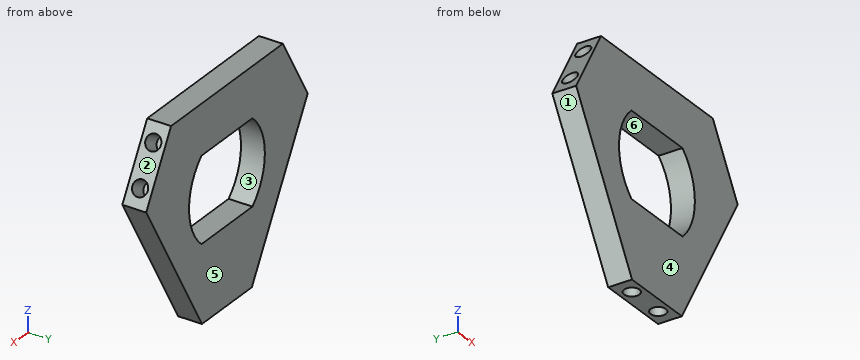
```python
from build123d import *

# Parameters (mm, degrees)
CROQUIS1_W              = 57.5
CROQUIS1_H              = 42.5
SALIENTE_EXTRUIR1_DEPTH = 12
CROQUIS7_R              = 46.25
CROQUIS7_R_2            = 28.75
SALIENTE_EXTRUIR2_DEPTH = 12
CROQUIS8_R              = 3.875
CORTAR_EXTRUIR1_DEPTH   = 10
MATRIZC1_COUNT          = 3


with BuildPart() as part:
    # Croquis1 → Saliente-Extruir1 (new body)
    with BuildSketch(Plane(origin=(0, 0, 0), x_dir=(1, 0, 0), z_dir=(0, 1, 0))):
        Polygon((-18.886751346, 59.787187079), (-61.220598504, -13.537187079), (-42.333847158, -46.25), (42.333847158, -46.25), (61.220598504, -13.537187079), (18.886751346, 59.787187079), align=None)
        Rectangle(CROQUIS1_W, CROQUIS1_H, mode=Mode.SUBTRACT)
    extrude(amount=SALIENTE_EXTRUIR1_DEPTH)

    # Croquis7 → Saliente-Extruir2 (add)
    with BuildSketch(Plane(origin=(0, 0, 0), x_dir=(1, 0, 0), z_dir=(0, 1, 0))):
        Circle(CROQUIS7_R)
        Circle(CROQUIS7_R_2, mode=Mode.SUBTRACT)
    extrude(amount=SALIENTE_EXTRUIR2_DEPTH)

    # Croquis8 → Cortar-Extruir1 (cut)
    with BuildSketch(Plane(origin=(51.777222831, 0, 29.893593539), x_dir=(0.5, 0, -0.866025404), z_dir=(0.866025404, 0, 0.5))):
        with Locations((-10, 6)):
            Circle(CROQUIS8_R)
        with Locations((10, 6)):
            Circle(CROQUIS8_R)
    cortar_extruir1 = extrude(amount=-CORTAR_EXTRUIR1_DEPTH, mode=Mode.SUBTRACT)

    # MatrizC1: Cortar-Extruir1 ×3 about axis
    matrizc1_axis = Axis((0, 0, 0), (0, 1, 0))
    for i in range(1, MATRIZC1_COUNT):
        add(cortar_extruir1.rotate(matrizc1_axis, i * 360 / MATRIZC1_COUNT), mode=Mode.SUBTRACT)


solid = part.part
```
Geometry check sheet. Reference: the model listing, model coordinates, mm. Face numbers are marked on the shaded views. A direction names the side the tool comes from. Coordinates: 2 decimals unless noted, no trailing zeros. Order: outer loops, then holes, each group sorted by start corner. A loop starts at its lowest first (then second) coordinate and runs counter-clockwise, first axis right, second up.
Q1. Depth check by flat-ended pin: pin 1 Ø6 at (y, z) = (6, 19) entering from -X; pin 2 Ø4 at (x, y) = (11.5, 5.5) entering from -Z; pin 3 Ø6 at (y, z) = (10, -7.5) entering from -X. Enter the tip coordinate at first touch or a pass-through.
Reply:
pin 1: stops at x = -59.8
pin 2: stops at z = -49.79
pin 3: stops at x = -50.81
Q2. Sectioned sample at D-D on x = -26. Record the cut outline in (y, z).
Reply:
outline: (0, -47.47) - (12, -47.47) - (12, -12.27) - (0, -12.27) - close; (0, 12.27) - (12, 12.27) - (12, 46.25) - (0, 46.25) - close
Q3. Thickness scan on probe 1 along Z at (x, y) = (4, 7.75); probe 2 along Z at (x, y) = (-13, 7); probe 3 along Z at (x, y) = (-32.5, 9). Record the ranges inside material, lowest first.
Reply:
probe 1: z = -59.79 to -21.25, 21.25 to 46.25
probe 2: z = -49.79 to -21.25, 21.25 to 46.25
probe 3: z = -36.21 to 46.25
Q4. Tool access check on the marked faces 5 and 6. Record the directions out of +Z, -Z, +X, -X, +Y, -Y that give a thin tool (end or side, any length) a straight path to the whole face; none if there is none.
Reply:
face 5: +Z, -Z, +X, -X, +Y
face 6: +Y, -Y
Q5. Sectioned sample at B-B on z = 1. Record the cut outline in (x, y), and give its area (3 significant figures).
Reply:
outline: (-53.98, 0) - (-28.73, 0) - (-28.73, 12) - (-53.98, 12) - close; (28.73, 0) - (53.98, 0) - (53.98, 12) - (28.73, 12) - close
area: 606 mm2
Q6. Sectioned sample at A-A on x = -10. Record the cut outline in (y, z) (3 decimals).
Reply:
outline: (0, -59.787) - (2.125, -59.787) - (2.125, -49.787) - (9.875, -49.787) - (9.875, -59.787) - (12, -59.787) - (12, -21.25) - (0, -21.25) - close; (0, 21.25) - (12, 21.25) - (12, 46.25) - (0, 46.25) - close
Q7. Draft check along X on the marked faces 1, 2, 3 and 4. Enter one of: released by +X, released by -X, zero draft, split by the parting line, or undercut.
Reply:
face 1: released by -X
face 2: released by +X
face 3: undercut
face 4: zero draft
